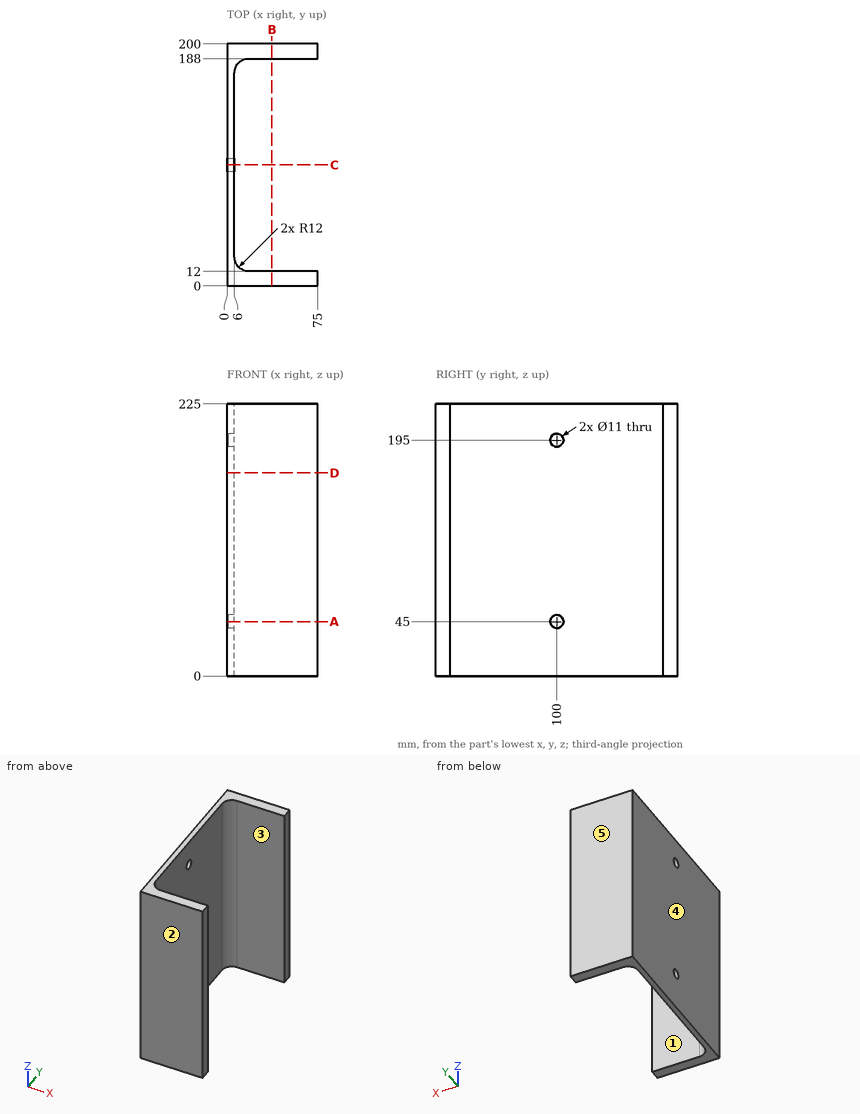
Answer from the drawing. Dimensions are ordinates in mm from the lowest x, y and z of the part. A direction names the side the tool comes from. Give positions to 0.01 mm unless a question says otherwise; leave off trailing zeros. Loops run counter-clockwise (first coordinate to the right, second up) from the corner with the lowest first, then second, coordinate; pieces in that order, holes last.
Item 1: A cutting plane is placed at A-A (z = 45). Give the vertices of the cut face in (x, y).
Derived:
outline: (0, 0) - (75, 0) - (75, 12) - (18, 12) arc R12 cw to (6, 24) - (6, 94.5) - (0, 94.5) - close; (0, 105.5) - (6, 105.5) - (6, 176) arc R12 cw to (18, 188) - (75, 188) - (75, 200) - (0, 200) - close
Item 2: Find the intervals of material crossed by line 1 along Z through (x, y) = (1, 100); line 2 along Y through (x, z) = (71.5, 173); line 3 along Y through (x, z) = (4.7, 195), in increasing order.
Derived:
line 1: z = 0 to 39.5, 50.5 to 189.5, 200.5 to 225
line 2: y = 0 to 12, 188 to 200
line 3: y = 0 to 94.5, 105.5 to 200
Item 3: A cutting plane is placed at B-B (x = 37). Give the vertices of the cut face in (y, z), then the cut area to 3 significant figures.
Derived:
outline: (0, 0) - (12, 0) - (12, 225) - (0, 225) - close; (188, 0) - (200, 0) - (200, 225) - (188, 225) - close
area: 5,400 mm2
Item 4: A tool of negligible diameter and unlimited length cuts with its end or side. For the marked faces 1 and 2, from which of +Z, -Z, +X, -X, +Y, -Y can it reach the whole face along a straight path? Write none if from no direction.
Derived:
face 1: +Z, -Z, +X
face 2: +Z, -Z, +X, -X, -Y
Item 5: A cutting plane is placed at D-D (z = 168). Give the vertices of the cut face in (x, y), then the cut area to 3 significant figures.
Derived:
outline: (0, 0) - (75, 0) - (75, 12) - (18, 12) arc R12 cw to (6, 24) - (6, 176) arc R12 cw to (18, 188) - (75, 188) - (75, 200) - (0, 200) - close
area: 2,920 mm2
Item 6: This flat-tipped pin is pushed along its axis until it touches: pin 1 Ø12.5 at (y, z) = (100, 195) entering from +X. Where does it stop, or does it pass through?
Derived:
pin 1: stops at x = 6
Item 7: A cutting plane is placed at C-C (y = 100). Give the vertices of the cut face in (x, z).
Derived:
outline: (0, 0) - (6, 0) - (6, 39.5) - (0, 39.5) - close; (0, 50.5) - (6, 50.5) - (6, 189.5) - (0, 189.5) - close; (0, 200.5) - (6, 200.5) - (6, 225) - (0, 225) - close
Item 8: Determine the mould class of the marked faces 3, 4 and 5 for opening direction Y: +Y half, -Y half, draft (parallel to the pull), parting line (faces both ways), or undercut.
Derived:
face 3: undercut
face 4: draft
face 5: +Y half
